Verification items for the finished model (mm, model axes). Give positions to 0.01 mm unless a question says otherwise; leave off trailing zeros. Order: outer loops, then holes, each group sorted by start corner. A loop starts at its lowest first (then second) coordinate and runs counter-clockwise, first axis right, second up.
(1) Sectioned sample at C-C on x = 24.5. Record the cut outline in (y, z), plus the area to 3 significant figures.
(2) Scan lines: L1, parallel to Y at x = 0, z = -4.05; L2, parallel to Y at x = 167.5, z = -4.55; L3, parallel to Y at x = 14, z = -1.85. Record each from-to range of solid material in increasing order.
(3) Gauge pin test, flat end, axial feed: pin 1 (1.5 mm diameter, centred on y = 32.5, z = -1, fed in from +X). Record the tip position at first contact, or that the pin passes through.
(4) Sectioned sample at A-A on z = -3.95. Record the cut outline in (x, y).
(5) Sectioned sample at B-B on x = 294.5. Record the cut outline in (y, z), plus the area to 3 significant figures.
(6) Mould release check, pull along X, two halves, no side actions. Record for faces 1 (the face through (-27.15, -41.99, -3.04)), 2 (the face through (1.172, 53.923, -3.042)), 3 (the face through (217, -11, -6)), 4 (the face through (466.99, -42.15, -3.04)): pulls with the +X half, pulls with the -X half, needs draft (parallel to the pull), parting line crosses it, or undercut.
```python
from build123d import *

# Parameters (mm, degrees)
SALIENTE_EXTRUIR1_DEPTH = 6
REDONDEO1_R             = 10
REDONDEO2_R             = 10
CROQUIS2_R              = 9
CORTAR_EXTRUIR1_DEPTH   = 476.984243437
CROQUIS3_R              = 1.5
CORTAR_EXTRUIR2_DEPTH   = 476.984243437


with BuildPart() as part:
    # Croquis1 → Saliente-Extruir1 (new body)
    with BuildSketch(Plane.XY):
        with BuildLine():
            Line((30, -45), (470, -45))
            Line((470, -45), (470, 15))
            Line((470, 15), (30, 15))
            Line((30, 15), (30, 45))
            ThreePointArc((30, 45), (0, 75), (-30, 45))
            Line((-30, 45), (-30, -45))
            Line((-30, -45), (30, -45))
        make_face()
    extrude(amount=-SALIENTE_EXTRUIR1_DEPTH)

    # Redondeo1
    redondeo1_edges = [part.edges().sort_by_distance(p)[0] for p in [
        (-30, -45, -3),
    ]]
    fillet(redondeo1_edges, radius=REDONDEO1_R)

    # Redondeo2
    redondeo2_edges = [part.edges().sort_by_distance(p)[0] for p in [
        (470, 15, -3),
        (470, -45, -3),
    ]]
    fillet(redondeo2_edges, radius=REDONDEO2_R)

    # Croquis2 → Cortar-Extruir1 (cut, through all)
    with BuildSketch(Plane(origin=(0, 0, -6), x_dir=(-1, 0, 0), z_dir=(0, 0, -1))):
        with Locations((0, 45)):
            Circle(CROQUIS2_R)
    extrude(amount=-CORTAR_EXTRUIR1_DEPTH, mode=Mode.SUBTRACT)

    # Croquis3 → Cortar-Extruir2 (cut, through all)
    with BuildSketch(Plane(origin=(0, 0, -6), x_dir=(-1, 0, 0), z_dir=(0, 0, -1))):
        with Locations((0, 31)):
            Circle(CROQUIS3_R)
        with Locations((14, 45)):
            Circle(CROQUIS3_R)
        with Locations((0, 59)):
            Circle(CROQUIS3_R)
        with Locations((-14, 45)):
            Circle(CROQUIS3_R)
    extrude(amount=-CORTAR_EXTRUIR2_DEPTH, mode=Mode.SUBTRACT)


solid = part.part
```
Ans:
1. outline: (-45, -6) - (62.31, -6) - (62.31, 0) - (-45, 0) - close
1. area: 644 mm2
2. L1: y = -45 to 29.5, 32.5 to 36, 54 to 57.5, 60.5 to 75
2. L2: y = -45 to 15
2. L3: y = -45 to 43.5, 46.5 to 71.53
3. pin 1: stops at x = 30
4. outline: (-30, -35) arc R10 ccw to (-20, -45) - (460, -45) arc R10 ccw to (470, -35) - (470, 5) arc R10 ccw to (460, 15) - (30, 15) - (30, 45) arc R30 ccw to (-30, 45) - close; hole circle Ø3 at (-14, 45); hole circle Ø18 at (0, 45); hole circle Ø3 at (0, 31); hole circle Ø3 at (0, 59); hole circle Ø3 at (14, 45)
5. outline: (-45, -6) - (15, -6) - (15, 0) - (-45, 0) - close
5. area: 360 mm2
6. face 1: pulls with the -X half
6. face 2: undercut
6. face 3: needs draft
6. face 4: pulls with the +X half
